```python
from build123d import *

# Parameters (mm, degrees)
PAD008_DEPTH    = 3
POCKET011_DEPTH = 5
SKETCH043_R     = 1.45
POCKET017_DEPTH = 22
POCKET023_DEPTH = 28
SKETCH059_R     = 0.15
POCKET030_DEPTH = 32
FILLET006_R     = 1.5
FILLET014_R     = 0.5


with BuildPart() as part:
    # Sketch030 → Pad008 (new body)
    with BuildSketch(Plane.XY):
        with BuildLine():
            Line((153.231854, -38.154949), (175.310198, 11.234895))
            add(Edge.make_bspline(
                [(150.875, 88.9625), (150.875, 42.8625), (150.875, 22.157965), (175.310198, 11.234895)],
                knots=[0, 0, 0, 0, 1, 1, 1, 1], degree=3))
            add(Edge.make_bspline(
                [(85.725, 98.4875), (104.775, 98.4875), (104.775, 88.9625), (150.875, 88.9625)],
                knots=[0, 0, 0, 0, 1, 1, 1, 1], degree=3))
            Line((85.725, 98.4875), (66.675, 98.4875))
            add(Edge.make_bspline(
                [(66.675, 98.4875), (45.641399, 98.334473), (40.615566, 90.142487), (20.066667, 86.427261)],
                knots=[0, 0, 0, 0, 1, 1, 1, 1], degree=3))
            Line((20.066667, 86.427261), (20.066667, -8.521476))
            add(Edge.make_bspline(
                [(20.066667, -8.521476), (32.593586, -9.362079), (39.625488, -11.778089), (39.625, -17.525)],
                knots=[0, 0, 0, 0, 1, 1, 1, 1], degree=3))
            add(Edge.make_bspline(
                [(153.231854, -38.154949), (107.082107, -17.525), (76.2, -17.525), (39.625, -17.525)],
                knots=[0, 0, 0, 0, 1, 1, 1, 1], degree=3))
        make_face()
    extrude(amount=PAD008_DEPTH)

    # Sketch031 → Pocket011 (cut)
    with BuildSketch(Plane(origin=(0, 0, 0), x_dir=(1, 0, 0), z_dir=(0, 0, -1))):
        Polygon((85.725, -86.475), (105.525, -86.475), (105.525, -81.7125), (143.625, -81.7125), (143.625, -17.457464), (165.732668, -7.574851), (149.57181, 28.577419), (131.568158, 20.529392), (102.96164, 14.448889), (103.848827, 10.275), (85.725, 10.275), align=None)
    extrude(amount=-POCKET011_DEPTH, mode=Mode.SUBTRACT)

    # Sketch043 → Pocket017 (cut)
    with BuildSketch(Plane.XY):
        with Locations((-4.375, -4.375)):
            Circle(SKETCH043_R)
        with Locations((-4.375, 80.575)):
            Circle(SKETCH043_R)
        with Locations((151.401832, -33.366184)):
            Circle(SKETCH043_R)
        with Locations((170.521433, 9.404873)):
            Circle(SKETCH043_R)
        with Locations((147.25, 85.3375)):
            Circle(SKETCH043_R)
        with Locations((43.25, -13.9)):
            Circle(SKETCH043_R)
        with Locations((57.15, 92.085)):
            Circle(SKETCH043_R)
        with Locations((95.25, 92.085)):
            Circle(SKETCH043_R)
        with Locations((95.25, -13.9)):
            Circle(SKETCH043_R)
    extrude(amount=POCKET017_DEPTH, mode=Mode.SUBTRACT)

    # Sketch051 → Pocket023 (cut)
    with BuildSketch(Plane.XY):
        Polygon((142.875, 69.9125), (142.875, 55.9125), (154.875, 54.9125), (154.875, 70.9125), align=None)
    extrude(amount=POCKET023_DEPTH, mode=Mode.SUBTRACT)

    # Sketch059 → Pocket030 (cut)
    with BuildSketch(Plane.XY):
        with Locations((134.25, 85.3375)):
            Circle(SKETCH059_R)
        with Locations((147.25, 74.3375)):
            Circle(SKETCH059_R)
    extrude(amount=POCKET030_DEPTH, mode=Mode.SUBTRACT)

    # Fillet006
    fillet006_edges = [part.edges().sort_by_distance(p)[0] for p in [
        (39.625, -17.525, 1.5),
        (153.231854, -38.154949, 1.5),
        (175.310198, 11.234895, 1.5),
        (150.875, 88.9625, 1.5),
    ]]
    fillet(fillet006_edges, radius=FILLET006_R)

    # Fillet014
    fillet014_edges = [part.edges().sort_by_distance(p)[0] for p in [
        (20.066667, -8.521476, 1.5),
        (20.066667, 86.427261, 1.5),
    ]]
    fillet(fillet014_edges, radius=FILLET014_R)


with BuildPart() as part_1:
    # Body007 placement: moved
    add(part.part.moved(Location((0, 0, -12))))


solid = part_1.part
```
Source: CAD feature listing. Evaluate the final solid. Frame: model axes, mm. A direction names the side the tool comes from. Coordinates: 2 decimals unless noted, no trailing zeros. Order: outer loops, then holes, each group sorted by start corner. A loop starts at its lowest first (then second) coordinate and runs counter-clockwise, first axis right, second up. Notation, with made-up numbers: M -12.75,86.5 L 10.25,86.5 A28 ccw 10.25,119.5 Z; hole C -3,17 d2. An arc over 180 degrees is marked long. Write each question's results on one line, items separated by ' | '. Start each with the question number.
1) Line query: line 1 (X direction, y = -13.9, z = -10.9); line 2 (Y direction, x = 147.25, z = -9.65); line 3 (X direction, y = 42, z = -10.8) (3 decimals). Output: solid intervals per line, ascending. Write a range as from..to.
2) Draft query along Y for faces 3 (the face through (117.465, -17.532, -10.521)), 4 (the face through (79, 31, -12)), 5 (the face through (164.13, -13.78, -10.52)). Return one class per face: released by +Y, released by -Y, zero draft, split by the parting line, or undercut.
3) Contact query for flat-ended pins moving along their axis: pin 1 Ø2.5 at (x, y) = (170.52, 9.4) entering from +Z; pin 2 Ø0.9 at (x, z) = (92.5, -11) entering from -Y. Output: stop coordinate, or through.
4) Section query A-A (y = 5). Return the cut outline in (x, z) (3 decimals).
5) Access query for faces 1 (the face through (79, 31, -9)), 2 (the face through (140.7, -24.61, -10.52)). Directions: +Z, -Z, +X, -X, +Y, -Y. A direction counts if a zero-diameter tool reaches every point of the face in a straight line with its end or side. Return the directions, or none.
6) Section query B-B (z = -10.3). Give the number of separate pieces and of enclosed holes in the cut face, plus the area to 3 significant figures.
Answers:
1) line 1: x = 38.4..41.8, 44.7..93.8, 96.7..103.08, 156.13..164.07 | line 2: y = -35.56..-27.54, 15.84..55.55, 70.28..74.19, 74.49..83.89, 86.79..88.98 | line 3: x = 20.067..85.725, 143.625..152.875
2) face 3: undercut | face 4: zero draft | face 5: released by -Y
3) pin 1: passes through | pin 2: stops at y = -20.12
4) outline: M 20.067,-12 L 85.725,-12 L 85.725,-9 L 20.067,-9 Z; M 164.582,-12 L 172.523,-12 L 172.523,-9 L 164.582,-9 Z
5) face 1: +Z, +X, -X, +Y, -Y | face 2: +Z, -Z
6) separate pieces: 1 | enclosed holes: 9 | area: 9,400 mm^2
